```python
from build123d import *

# Parameters (mm, degrees)
F0_R     = 1.63195
F1_DEPTH = 5
F2_W     = 35
F2_H     = 18.64
F3_DEPTH = 50
F5_DEPTH = 90.481


with BuildPart() as f1:
    # F0 (on Top) → F1 (new body)
    with BuildSketch(Plane.XY):
        Polygon((-52.48, 53.76), (-52.48, -53.76), (-3, -53.76), (-3, -41.76), (3, -41.76), (3, -53.76), (52.48, -53.76), (52.48, 53.76), align=None)
        with Locations((-48.73, -50.01)):
            Circle(F0_R, mode=Mode.SUBTRACT)
        with Locations((48.73, -50.01)):
            Circle(F0_R, mode=Mode.SUBTRACT)
        with Locations((-48.73, 50.01)):
            Circle(F0_R, mode=Mode.SUBTRACT)
        with Locations((48.73, 50.01)):
            Circle(F0_R, mode=Mode.SUBTRACT)
    extrude(amount=F1_DEPTH)

    # F2 (on face) → F3 (join)
    with BuildSketch(Plane.XY.offset(5)):
        with Locations((20.5, -44.44)):
            Rectangle(F2_W, F2_H)
        with Locations((-20.5, -44.44)):
            Rectangle(F2_W, F2_H)
    extrude(amount=-F3_DEPTH)

    # F4 (on face) → F5 (cut, through all)
    with BuildSketch(Plane(origin=(-38, 0, 0), x_dir=(0, -1, 0), z_dir=(-1, 0, 0))):
        Polygon((53.76, -45), (53.76, 0), (35.1203896932, -45), align=None)
    extrude(amount=-F5_DEPTH, mode=Mode.SUBTRACT)


solid = f1.part
```
Build history of the part. All positions in model axes, mm. A direction names the side the tool comes from. Round coordinates to 2 decimals unless told otherwise and drop trailing zeros. Order: outer loops, then holes, each group sorted by start corner. A loop starts at its lowest first (then second) coordinate and runs counter-clockwise, first axis right, second up. Notation, with made-up numbers: (77.25, 2) -> (119.25, 2) arc R27 ccw to (119.25, 23) -> close; hole circle Ø4 at (41, 52). An arc over 180 degrees is marked (long way). Answer in a Markdown table with one row per item.
1) Which spindle directions (+Z, -Z, +X, -X, +Y, -Y) get a long thin tool onto all of the face, cutting with end or side? Do faces 5 (the flat face through (-21, -35.12, -22)), 6 (the flat face through (3, -42, -14)), 7 (the flat face through (-38, -42, -17)), 8 (the cylindrical face through (48.376, 48.417, 2.465)). Say none if no direction does.
Values:
| item | result |
|---|---|
| face 5 | -Z, +X, -X, +Y |
| face 6 | -Z, -Y |
| face 7 | -Z, -X, +Y, -Y |
| face 8 | +Z, -Z |
2) Wall check: L1, parallel to Y at x = 48.73, z = 1.2; L2, parallel to X at y = -50, z = 1; L3, parallel to X at y = 50, z = 1. Give the ranges that are in metal, low to high.
Values:
| item | result |
|---|---|
| L1 | -53.76 to -51.64, -48.38 to 48.38, 51.64 to 53.76 |
| L2 | -52.48 to -50.36, -47.1 to -3, 3 to 47.1, 50.36 to 52.48 |
| L3 | -52.48 to -50.36, -47.1 to 47.1, 50.36 to 52.48 |
3) Band-saw the part on B-B on x = 48.73. Give the cut face in (y, z).
Values:
| item | result |
|---|---|
| outline | (-53.76, 0) -> (-51.64, 0) -> (-51.64, 5) -> (-53.76, 5) -> close; (-48.38, 0) -> (48.38, 0) -> (48.38, 5) -> (-48.38, 5) -> close; (51.64, 0) -> (53.76, 0) -> (53.76, 5) -> (51.64, 5) -> close |
4) Mould opens along Y. For faces 1 (the flat face through (52.48, -1, 2)), 2 (the cylindrical face through (-50.025, 49.017, 2.465)), 3 (the flat face through (0, -41.76, 2)), 4 (the cylindrical face through (48.376, -51.603, 2.465)) say: released by +Y, released by -Y, zero draft, split by the parting line, or undercut.
Values:
| item | result |
|---|---|
| face 1 | zero draft |
| face 2 | undercut |
| face 3 | released by -Y |
| face 4 | undercut |
5) Pin check, flat tips, straight feed: P1, Ø10.5, axis at x = -29, z = -13, coming from the +Y side; P2, Ø15, axis at y = -46, z = -29.5, coming from the -X side; P3, Ø4, axis at x = 48.73, y = -50.01, coming from the -Z side; P4, Ø3, axis at x = -48.73, y = -50.01, coming from the +Z side. Stop position of each tip, or through.
Values:
| item | result |
|---|---|
| P1 | y = -35.12 |
| P2 | x = -38 |
| P3 | z = 0 |
| P4 | through |
6) Band-saw the part on D-D on y = -50.01. Give the cut face in (x, z), and give its area (3 significant figures).
Values:
| item | result |
|---|---|
| outline | (-52.48, 0) -> (-50.36, 0) -> (-50.36, 5) -> (-52.48, 5) -> close; (-47.1, 0) -> (-38, 0) -> (-38, -9.05) -> (-3, -9.05) -> (-3, 5) -> (-47.1, 5) -> close; (3, -9.05) -> (38, -9.05) -> (38, 0) -> (47.1, 0) -> (47.1, 5) -> (3, 5) -> close; (50.36, 0) -> (52.48, 0) -> (52.48, 5) -> (50.36, 5) -> close |
| area | 1,100 mm2 |
7) Band-saw the part on C-C on z = -25.5. Give the cut face in (x, y).
Values:
| item | result |
|---|---|
| outline | (-38, -43.2) -> (-3, -43.2) -> (-3, -35.12) -> (-38, -35.12) -> close; (3, -43.2) -> (38, -43.2) -> (38, -35.12) -> (3, -35.12) -> close |
8) Band-saw the part on A-A on y = 50.01. Give the cut face in (x, z), and give its area (3 significant figures).
Values:
| item | result |
|---|---|
| outline | (-52.48, 0) -> (-50.36, 0) -> (-50.36, 5) -> (-52.48, 5) -> close; (-47.1, 0) -> (47.1, 0) -> (47.1, 5) -> (-47.1, 5) -> close; (50.36, 0) -> (52.48, 0) -> (52.48, 5) -> (50.36, 5) -> close |
| area | 492 mm2 |
